Geometry: final body of the model. Coordinates: model frame, mm. Face numbers are marked on the shaded views. A direction names the side the tool comes from. Round coordinates to 2 decimals unless told otherwise and drop trailing zeros. Loops run counter-clockwise (first coordinate to the right, second up) from the corner with the lowest first, then second, coordinate; pieces in that order, holes last. Notation, with made-up numbers: M 58,74.5 L 73,74.5 A27 ccw 73,91.5 Z; hole C 53.25,57.5 d2. An arc over 180 degrees is marked long. Answer as a JSON object with one key per item and string values.
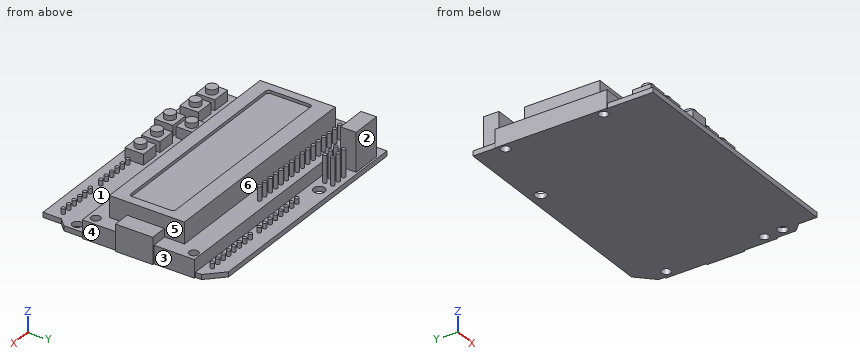
```python
from build123d import *

# Parameters (mm, degrees)
SKETCH2_W            = 71.12
SKETCH2_H            = 24.13
BOSS_EXTRUDE1_DEPTH  = 12.63
SKETCH3_W            = 80.5
SKETCH3_H            = 36
SKETCH3_R            = 1.4859
BOSS_EXTRUDE2_DEPTH  = 5.8
SKETCH4_R            = 1.8288
SKETCH4_R_2          = 1.6
SKETCH4_R_3          = 1.4859
BOSS_EXTRUDE4_DEPTH  = 1.6
SKETCH5_R            = 1.75
BOSS_EXTRUDE5_DEPTH  = 6.6
SKETCH6_W            = 6
SKETCH6_H            = 6
BOSS_EXTRUDE6_DEPTH  = 5
SKETCH7_W            = 9.6
SKETCH7_H            = 5
BOSS_EXTRUDE7_DEPTH  = 14
SKETCH8_R            = 0.607588519
BOSS_EXTRUDE8_DEPTH  = 10.3
SKETCH9_R            = 0.6
BOSS_EXTRUDE9_DEPTH  = 3.3
SKETCH10_R           = 0.6
BOSS_EXTRUDE10_DEPTH = 10.3
SKETCH11_W           = 5.5
SKETCH11_H           = 12
BOSS_EXTRUDE11_DEPTH = 8.5
CUT_EXTRUDE1_DEPTH   = 1


with BuildPart() as part:
    # Sketch2 → Boss-Extrude1 (new body)
    with BuildSketch(Plane.XY):
        with Locations((39.392131734, 32.008259463)):
            Rectangle(SKETCH2_W, SKETCH2_H)
    extrude(amount=BOSS_EXTRUDE1_DEPTH)

    # Sketch3 → Boss-Extrude2 (add)
    with BuildSketch(Plane.XY):
        with Locations((39.764131734, 32.677259463)):
            Rectangle(SKETCH3_W, SKETCH3_H)
        with Locations((1.524412377, 48.661369793)):
            Circle(SKETCH3_R, mode=Mode.SUBTRACT)
        with Locations((1.524412377, 17.153759759)):
            Circle(SKETCH3_R, mode=Mode.SUBTRACT)
        with Locations((77.309031734, 17.153759463)):
            Circle(SKETCH3_R, mode=Mode.SUBTRACT)
        with Locations((77.309031734, 48.661369497)):
            Circle(SKETCH3_R, mode=Mode.SUBTRACT)
    extrude(amount=BOSS_EXTRUDE2_DEPTH)

    # Sketch4 → Boss-Extrude4 (add)
    with BuildSketch(Plane.XY):
        Polygon((-0.342397773, 57.8612), (74.3712, 57.8612), (79.5528, 52.6796), (79.5528, 8.4836), (77.0128, 5.880101811), (77.0128, 0), (-0.342397773, 0), align=None)
        with Locations((26.2128, 54.2036)):
            Circle(SKETCH4_R, mode=Mode.SUBTRACT)
        with Locations((77.0128, 11.0236)):
            Circle(SKETCH4_R_2, mode=Mode.SUBTRACT)
        with Locations((1.524412377, 48.661369793)):
            Circle(SKETCH4_R_3, mode=Mode.SUBTRACT)
        with Locations((1.524412377, 17.153759759)):
            Circle(SKETCH4_R_3, mode=Mode.SUBTRACT)
        with Locations((77.309031734, 17.153759463)):
            Circle(SKETCH4_R_3, mode=Mode.SUBTRACT)
        with Locations((77.309031734, 48.661369497)):
            Circle(SKETCH4_R_3, mode=Mode.SUBTRACT)
    extrude(amount=BOSS_EXTRUDE4_DEPTH)

    # Sketch5 → Boss-Extrude5 (add)
    with BuildSketch(Plane.XY):
        with Locations(Location((5.460845243, 5.527822186, 0), (0, 0, 180))):
            Circle(SKETCH5_R)
        with Locations(Location((39.115845243, 5.527822186, 0), (0, 0, 180))):
            Circle(SKETCH5_R)
        with Locations(Location((31.368845243, 5.527822186, 0), (0, 0, 180))):
            Circle(SKETCH5_R)
        with Locations(Location((22.537232927, 3.6978, 0), (0, 0, 180))):
            Circle(SKETCH5_R)
        with Locations(Location((22.537232927, 10.6828, 0), (0, 0, 180))):
            Circle(SKETCH5_R)
        with Locations(Location((13.207845243, 5.527822186, 0), (0, 0, 180))):
            Circle(SKETCH5_R)
    extrude(amount=BOSS_EXTRUDE5_DEPTH)

    # Sketch6 → Boss-Extrude6 (add)
    with BuildSketch(Plane.XY):
        with Locations((5.460845243, 5.527822186)):
            Rectangle(SKETCH6_W, SKETCH6_H)
        with Locations((13.207845243, 5.527822186)):
            Rectangle(SKETCH6_W, SKETCH6_H)
        with Locations((22.537232927, 10.6828)):
            Rectangle(SKETCH6_W, SKETCH6_H)
        with Locations((22.537232927, 3.6978)):
            Rectangle(SKETCH6_W, SKETCH6_H)
        with Locations((31.368845243, 5.527822186)):
            Rectangle(SKETCH6_W, SKETCH6_H)
        with Locations((39.115845243, 5.527822186)):
            Rectangle(SKETCH6_W, SKETCH6_H)
    extrude(amount=BOSS_EXTRUDE6_DEPTH)

    # Sketch7 → Boss-Extrude7 (add)
    with BuildSketch(Plane.XY):
        with Locations((8.4674, 54.729)):
            Rectangle(SKETCH7_W, SKETCH7_H)
    extrude(amount=BOSS_EXTRUDE7_DEPTH)

    # Sketch8 → Boss-Extrude8 (add)
    with BuildSketch(Plane.XY):
        with Locations((45.183190385, 47.927259463)):
            Circle(SKETCH8_R)
        with Locations((42.655890385, 47.927259463)):
            Circle(SKETCH8_R)
        with Locations((40.128590385, 47.927259463)):
            Circle(SKETCH8_R)
        with Locations((37.601290385, 47.927259463)):
            Circle(SKETCH8_R)
        with Locations((35.073990385, 47.927259463)):
            Circle(SKETCH8_R)
        with Locations((32.546690385, 47.927259463)):
            Circle(SKETCH8_R)
        with Locations((30.019390385, 47.927259463)):
            Circle(SKETCH8_R)
        with Locations((27.492090385, 47.927259463)):
            Circle(SKETCH8_R)
        with Locations((24.964790385, 47.927259463)):
            Circle(SKETCH8_R)
        with Locations((22.437490385, 47.927259463)):
            Circle(SKETCH8_R)
        with Locations((19.910190385, 47.927259463)):
            Circle(SKETCH8_R)
        with Locations((17.382890385, 47.927259463)):
            Circle(SKETCH8_R)
        with Locations((14.855590385, 47.927259463)):
            Circle(SKETCH8_R)
        with Locations((12.328290385, 47.927259463)):
            Circle(SKETCH8_R)
        with Locations((9.800990385, 47.927259463)):
            Circle(SKETCH8_R)
        with Locations((7.273690385, 47.927259463)):
            Circle(SKETCH8_R)
    extrude(amount=BOSS_EXTRUDE8_DEPTH)

    # Sketch9 → Boss-Extrude9 (add)
    with BuildSketch(Plane.XY):
        with Locations(Location((74.399505323, 4.775685088, 0), (0, 0, 180))):
            Circle(SKETCH9_R)
        with Locations(Location((71.859505323, 4.775685088, 0), (0, 0, 180))):
            Circle(SKETCH9_R)
        with Locations(Location((69.319505323, 4.775685088, 0), (0, 0, 180))):
            Circle(SKETCH9_R)
        with Locations(Location((66.779505323, 4.775685088, 0), (0, 0, 180))):
            Circle(SKETCH9_R)
        with Locations(Location((64.239505323, 4.775685088, 0), (0, 0, 180))):
            Circle(SKETCH9_R)
        with Locations(Location((61.699505323, 4.775685088, 0), (0, 0, 180))):
            Circle(SKETCH9_R)
        with Locations(Location((56.696852257, 4.775685088, 0), (0, 0, 180))):
            Circle(SKETCH9_R)
        with Locations(Location((54.156852257, 4.775685088, 0), (0, 0, 180))):
            Circle(SKETCH9_R)
        with Locations(Location((51.616852257, 4.775685088, 0), (0, 0, 180))):
            Circle(SKETCH9_R)
        with Locations(Location((49.076852257, 4.775685088, 0), (0, 0, 180))):
            Circle(SKETCH9_R)
        with Locations(Location((46.536852257, 4.775685088, 0), (0, 0, 180))):
            Circle(SKETCH9_R)
        with Locations(Location((43.996852257, 4.775685088, 0), (0, 0, 180))):
            Circle(SKETCH9_R)
        with Locations(Location((75.037059203, 53.119768804, 0), (0, 0, 180))):
            Circle(SKETCH9_R)
        with Locations(Location((72.497059203, 53.119768804, 0), (0, 0, 180))):
            Circle(SKETCH9_R)
        with Locations(Location((69.957059203, 53.119768804, 0), (0, 0, 180))):
            Circle(SKETCH9_R)
        with Locations(Location((67.417059203, 53.119768804, 0), (0, 0, 180))):
            Circle(SKETCH9_R)
        with Locations(Location((64.877059203, 53.119768804, 0), (0, 0, 180))):
            Circle(SKETCH9_R)
        with Locations(Location((62.337059203, 53.119768804, 0), (0, 0, 180))):
            Circle(SKETCH9_R)
        with Locations(Location((59.797059203, 53.119768804, 0), (0, 0, 180))):
            Circle(SKETCH9_R)
        with Locations(Location((57.257059203, 53.119768804, 0), (0, 0, 180))):
            Circle(SKETCH9_R)
        with Locations(Location((52.939059203, 53.119768804, 0), (0, 0, 180))):
            Circle(SKETCH9_R)
        with Locations(Location((50.399059203, 53.119768804, 0), (0, 0, 180))):
            Circle(SKETCH9_R)
        with Locations(Location((47.859059203, 53.119768804, 0), (0, 0, 180))):
            Circle(SKETCH9_R)
        with Locations(Location((45.319059203, 53.119768804, 0), (0, 0, 180))):
            Circle(SKETCH9_R)
        with Locations(Location((42.779059203, 53.119768804, 0), (0, 0, 180))):
            Circle(SKETCH9_R)
        with Locations(Location((40.239059203, 53.119768804, 0), (0, 0, 180))):
            Circle(SKETCH9_R)
        with Locations(Location((37.699059203, 53.119768804, 0), (0, 0, 180))):
            Circle(SKETCH9_R)
        with Locations(Location((35.159059203, 53.119768804, 0), (0, 0, 180))):
            Circle(SKETCH9_R)
    extrude(amount=BOSS_EXTRUDE9_DEPTH)

    # Sketch10 → Boss-Extrude10 (add)
    with BuildSketch(Plane.XY):
        with Locations(Location((17.057745163, 53.220149318, 0), (0, 0, 180))):
            Circle(SKETCH10_R)
        with Locations(Location((19.597745163, 53.220149318, 0), (0, 0, 180))):
            Circle(SKETCH10_R)
        with Locations(Location((22.137745163, 53.220149318, 0), (0, 0, 180))):
            Circle(SKETCH10_R)
        with Locations(Location((22.137745163, 55.760149318, 0), (0, 0, 180))):
            Circle(SKETCH10_R)
        with Locations(Location((19.597745163, 55.760149318, 0), (0, 0, 180))):
            Circle(SKETCH10_R)
        with Locations(Location((17.057745163, 55.760149318, 0), (0, 0, 180))):
            Circle(SKETCH10_R)
    extrude(amount=BOSS_EXTRUDE10_DEPTH)

    # Sketch11 → Boss-Extrude11 (add)
    with BuildSketch(Plane.XY):
        with Locations((77.764131734, 31.677259463)):
            Rectangle(SKETCH11_W, SKETCH11_H)
    extrude(amount=BOSS_EXTRUDE11_DEPTH)

    # Sketch12 → Cut-Extrude1 (cut)
    with BuildSketch(Plane.XY.offset(12.63)):
        with BuildLine():
            Line((72.014131734, 25.177259463), (72.014131734, 37.677259463))
            ThreePointArc((72.014131734, 37.677259463), (71.721238515, 38.384366244), (71.014131734, 38.677259463))
            Line((71.014131734, 38.677259463), (7.514131734, 38.677259463))
            ThreePointArc((7.514131734, 38.677259463), (6.807024953, 38.384366244), (6.514131734, 37.677259463))
            Line((6.514131734, 37.677259463), (6.514131734, 25.177259463))
            ThreePointArc((6.514131734, 25.177259463), (6.807024953, 24.470152682), (7.514131734, 24.177259463))
            Line((7.514131734, 24.177259463), (71.014131734, 24.177259463))
            ThreePointArc((71.014131734, 24.177259463), (71.721238515, 24.470152682), (72.014131734, 25.177259463))
        make_face()
    extrude(amount=-CUT_EXTRUDE1_DEPTH, mode=Mode.SUBTRACT)


solid = part.part
```
1) Line query: probe 1 along X at (y, z) = (7.5, 3.75); probe 2 along Y at (x, z) = (19.5, 2.5); probe 3 along Y at (x, z) = (6.5, 11.5). Output: solid intervals per line, ascending.
Geometry results:
{"probe 1": "2.46 to 8.46, 10.21 to 16.21, 28.37 to 34.37, 36.12 to 42.12", "probe 2": "14.68 to 50.68, 52.63 to 53.81, 55.17 to 56.35", "probe 3": "19.94 to 44.07, 52.23 to 57.23"}
2) Set-up query: the marked faces 1, 2 and 3. Return all of +Z, -Z, +X, -X, +Y, -Y with unobstructed straight access to the full face (end or side cutting, diameter ignored); none if empty.
Geometry results:
{"face 1": "+Z", "face 2": "+Z, +X, -X, +Y", "face 3": "+Z, -Z, +X, +Y"}
3) Pull-direction query (X, two-part tool) for the marked faces 4, 5 and 6; classes: +X half, -X half, draft (parallel to the pull), parting line (faces both ways), or undercut.
Geometry results:
{"face 4": "+X half", "face 5": "undercut", "face 6": "draft"}
4) Cut plane A-A on y = 35. Return the cut outline in (x, z), and give its area (3 significant figures).
Geometry results:
{"outline": "M -0.49,0 L 80.51,0 L 80.51,8.5 L 75.01,8.5 L 75.01,5.8 L 74.95,5.8 L 74.95,12.63 L 72.01,12.63 L 72.01,11.63 L 6.51,11.63 L 6.51,12.63 L 3.83,12.63 L 3.83,5.8 L -0.49,5.8 Z", "area": "905 mm2"}
5) Cut plane B-B on y = 22. Return the cut outline in (x, z).
Geometry results:
{"outline": "M -0.49,0 L 80.01,0 L 80.01,5.8 L 74.95,5.8 L 74.95,12.63 L 3.83,12.63 L 3.83,5.8 L -0.49,5.8 Z"}
6) First-contact query: pin 1 (0.6 mm diameter, centred on x = 37.5, y = 53, fed in from +Z); pin 2 (5 mm diameter, centred on x = 1.52, y = 48.66, fed in from +Z); pin 3 (1.8 mm diameter, centred on x = 12.5, y = 4, fed in from +Z). Flat tips, straight axial feed; report the tip coordinate or a pass-through.
Geometry results:
{"pin 1": "z = 3.3", "pin 2": "z = 5.8", "pin 3": "z = 6.6"}
